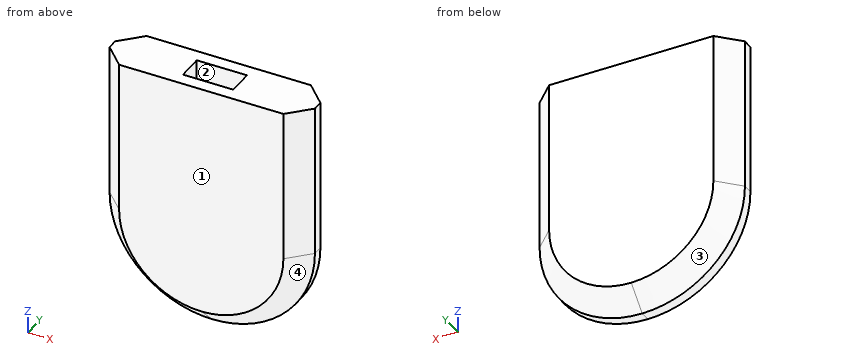
from build123d import *

# Parameters (mm, degrees)
F0_W     = 50.8
F0_H     = 12.7
F1_DEPTH = 25.4
F2_DEPTH = 63.5
F3_R     = 25.39999
F4_SIZE  = 5.08
F5_W     = 12.446
F5_H     = 6.35
F6_DEPTH = 25.4


# Not quite as in the source:
# - a fillet or chamfer is up to 0.001 mm smaller than in the source, because OpenCascade refuses the exact size


with BuildPart() as f1:
    # F0 (on Top) → F1 (new body)
    with BuildSketch(Plane.XY):
        Rectangle(F0_W, F0_H)
    extrude(amount=F1_DEPTH)

    # F0 (on Top) → F2 (join)
    with BuildSketch(Plane.XY):
        Rectangle(F0_W, F0_H)
    extrude(amount=F2_DEPTH)

    # F3 (radius 25.4 in the source; OpenCascade refuses exactly that, so slightly less here)
    f3_edges = [f1.edges().sort_by_distance(p)[0] for p in [
        (25.4, 0, 0),
        (-25.4, 0, 0),
    ]]
    fillet(f3_edges, radius=F3_R)

    # F4
    f4_edges = [f1.edges().sort_by_distance(p)[0] for p in [
        (-17.960515, -6.35, 7.439485),
        (-17.960515, 6.35, 7.439485),
    ]]
    chamfer(f4_edges, length=F4_SIZE)

    # F5 (on face) → F6 (cut)
    with BuildSketch(Plane.XY.offset(63.5)):
        Rectangle(F5_W, F5_H)
    extrude(amount=-F6_DEPTH, mode=Mode.SUBTRACT)


solid = f1.part
Here's how the part is built. I have some questions about the finished solid (model axes, mm). Face numbers are marked on the shaded views. Give positions to 0.01 mm unless a question says otherwise; leave off trailing zeros. Write each loop counter-clockwise with the first axis right and the second up, starting at its lowest first coordinate (ties: lowest second). Pieces come first, ordered by that corner, then holes. Notation, with made-up numbers: (47, 70.5) -> (90, 70.5) arc R21 cw to (90, 101.5) -> close; hole circle Ø2 at (-34, 62.5). An arc over 180 degrees is marked (long way). Use one line per item in the form item = value. Start each with the question number.
1. If I drill on L1, parallel to X at y = -1.5, z = 43.5; L2, parallel to Z at x = -11, y = 1.75; L3, parallel to X at y = 4.75, z = 11, over which ranges is the centre line in solid material (lowest first)?
2. Imagine slicing it at A-A on z = 44. List the corners of the cut face in (x, y) for me (3 decimals), plus the area to 3 significant figures.
3. Will these pins go through, and if not, where does the flat tip stop? pin 1 Ø1 at (y, z) = (-3, 8.5) entering from +X; pin 2 Ø6 at (y, z) = (3.5, 39.5) entering from +X; pin 3 Ø2 at (x, y) = (-10.5, -1) entering from -Z.
4. Thinking about a two-plate mould opening in X: for the marked faces 1, 2, 3 and 4, which applies, +X half, -X half, draft (parallel to the pull), parting line (faces both ways), or undercut?
5. Imagine slicing it at C-C on z = 32. List the corners of the cut face in (x, y) for me.
Entries:
q1.L1 = -25.17 to -6.22, 6.22 to 25.17
q1.L2 = 3.04 to 63.5
q1.L3 = -16.53 to 16.53
q2.outline = (-25.4, -1.27) -> (-20.32, -6.35) -> (20.32, -6.35) -> (25.4, -1.27) -> (25.4, 1.27) -> (20.32, 6.35) -> (-20.32, 6.35) -> (-25.4, 1.27) -> close; hole (-6.223, -3.175) -> (6.223, -3.175) -> (6.223, 3.175) -> (-6.223, 3.175) -> close
q2.area = 515 mm²
q3.pin_1 = 17.43
q3.pin_2 = 25.4
q3.pin_3 = 1.84
q4.face_1 = draft
q4.face_2 = undercut
q4.face_3 = -X half
q4.face_4 = +X half
q5.outline = (-25.4, -1.27) -> (-20.32, -6.35) -> (20.32, -6.35) -> (25.4, -1.27) -> (25.4, 1.27) -> (20.32, 6.35) -> (-20.32, 6.35) -> (-25.4, 1.27) -> close
